Autodesk Inventor part; units mm, degrees
ref_plane "Work Plane1" through (-0.254, 8.163, 9.525) normal (-1, 0, 0) x (0, 0, 1)
ref_plane "YZ Plane" through (0, 0, 0) normal (1, 0, 0) x (0, 1, 0)
ref_plane "XZ Plane" through (0, 0, 0) normal (0, 1, 0) x (-1, 0, 0)
sketch "Sketch1" plane through (0, 0, 0) normal (0, 0, 1) x (1, 0, 0)
  line L0 (0, 0) -> (66.675, 0)
  line L1 (66.675, 0) -> (66.675, 12.9255)
  line L2 (66.675, 12.9255) -> (0, 12.9255)
  line L3 (0, 12.9255) -> (0, 0)
  line L4 (66.675, 12.9255) -> (47.625, 12.9255)
  line L5 (47.625, 12.9255) -> (47.625, -23.7521)
  line L6 (47.625, -23.7521) -> (66.675, -23.7521)
  line L7 (66.675, -23.7521) -> (66.675, 12.9255)
  point P0 (57.15, -14.2271)
  point P1 (34.4424, 12.9255)
  point P2 (9.0424, 12.9255)
  dimension "d0" = 66.675
  dimension "d3" = 25.4
  dimension "d4" = 27.1526
  dimension "d5" = 0
  dimension "d41" = 48.1076
  dimension "d42" = 19.05
  dimension "d43" = 9.525
extrude "Extrusion1" add sketch "Sketch1" along normal blind 6.35
sketch "Sketch2" plane through (0, 0, 6.35) normal (0, 0, 1) x (1, 0, 0)
  line L0 (66.675, -23.7521) -> (66.675, 12.9255)
  line L1 (47.625, 0) -> (47.625, -23.7521)
  line L2 (66.675, 12.9255) -> (0, 12.9255)
  line L3 (47.625, -23.7521) -> (66.675, -23.7521)
  point P0 (0, 0)
  point P1 (57.15, -14.2271)
  dimension "d12" = 27.1526
  dimension "d44" = 9.525
  dimension "d45" = 9.525
  dimension "d46" = 9.525
hole "Hole1" at (57.15, -14.2271, 6.35) direction (0, 0, -1) diameter 6.25 depth 25.4 tip angle 118
sketch "Sketch3" plane through (0, 0, 6.35) normal (0, 0, 1) x (1, 0, 0)
  circle A0 centre (57.15, -14.2271) radius 3.125
  circle A1 centre (57.15, -14.2271) radius 9.525
  line L0 (47.625, -23.7521) -> (66.675, -23.7521)
  point P0 (0, 0)
extrude "Extrusion2" add sketch "Sketch3" along normal blind 12.7
fillet "Fillet1" radius 6.35 2 edges at (66.675, -23.7521, 3.175) (47.625, -23.7521, 3.175)
fillet "Fillet2" radius 25.4 2 edges at (47.625, 0, 3.175) (66.675, 12.9255, 3.175)
sketch "Sketch4" plane through (0, 0, 6.35) normal (0, 0, 1) x (1, 0, 0)
  line L0 (0, 12.9255) -> (0, 0)
  line L1 (0, 12.9255) -> (40.7924, 12.9255)
  line L2 (40.7924, 12.9255) -> (40.7924, 8.163)
  line L3 (40.7924, 8.163) -> (0, 8.163)
  line L4 (0, 8.163) -> (0, 12.9255)
  circle A0 centre (57.15, -14.2271) radius 3.125
  dimension "d24" = 16.3576
  dimension "d25" = 4.7625
extrude "Extrusion3" add sketch "Sketch4" along normal blind 9.525 contours L1 L2 L3 L0
fillet "Fillet3" radius 6.35 2 edges at (40.7924, 10.5443, 15.875) (0, 10.5443, 15.875)
fillet "Fillet4" radius 6.35 1 edges at (40.7924, 10.5443, 6.35)
sketch "Sketch5" plane through (6.35, 8.163, 15.875) normal (0, -1, 0) x (1, 0, 0)
  line L0 (47.675, 3.175) -> (53.925, 3.175)
  point P0 (-6.35, -15.875)
  point P1 (2.6924, -5.0739)
  point P2 (28.0924, -5.0739)
  point P3 (50.8, 3.175)
  dimension "d30" = 25.4
  dimension "d31" = 22.7076
hole "Hole2" at (9.0424, 8.163, 10.8011) at (34.4424, 8.163, 10.8011) at (57.15, 8.163, 19.05) direction (0, 1, 0) diameter 4.4958 depth 25.4 tip angle 118
fillet "Fillet5" radius 6.35 1 edges at (0, 0, 3.175)
fillet "Fillet6" radius 3.175 1 edges at (47.625, -14.2271, 19.05)
fillet "Fillet7" radius 3.175 1 edges at (54.025, -14.2271, 19.05)
ref_plane "Work Plane1" through (-0.254, 8.163, 9.525) normal (-1, 0, 0) x (0, 0, 1)
properties part number "supporty"
Check sheet for the modelled part. Datum: model origin and axes. Units: mm. A direction names the side the tool comes from. Round coordinates to 2 decimals unless told otherwise and drop trailing zeros. Write each loop counter-clockwise with the first axis right and the second up, starting at its lowest first coordinate (ties: lowest second). Pieces come first, ordered by that corner, then holes. Notation, with made-up numbers: (-14.75, 51) -> (7.25, 51) arc R22 cw to (7.25, 58) -> close; hole circle Ø5 at (58.25, 31.5). An arc over 180 degrees is marked (long way). One line per question, with ' | ' between items. Start each with the question number.
1. Scan lines: line 1 along Y through (x, z) = (57.15, 7); line 2 along X through (y, z) = (11.5, 11.5); line 3 along Z through (x, y) = (23, 5). Record each from-to range of solid material in increasing order. Write a range as from..to.
2. Depth check by flat-ended pin: pin 1 (4 mm diameter, centred on x = 15.5, y = 10, fed in from +Z) (3 decimals); pin 2 (1 mm diameter, centred on x = 30.5, y = 1.5, fed in from -Z); pin 3 (1.5 mm diameter, centred on x = 45.5, y = 3, fed in from +Z); pin 4 (4 mm diameter, centred on x = 34.44, z = 10.8, fed in from +Y). Enter the tip coordinate at first touch or a pass-through.
3. Release check for a two-part mould opening along Z. For faces 6 (the face through (32.55, 10.58, 9.59)), 7 (the face through (11.037, 10.578, 9.764)), 8 (the face through (38, 1, 6.35)), 9 (the face through (66.675, -15, 3)) record: +Z half, -Z half, draft (parallel to the pull), parting line (faces both ways), or undercut.
4. Sectioned sample at A-A, the plane z = 7. Count the separate pieces of the cut face and the enclosed holes in it, then the cut area to 3 significant figures.
5. Sectioned sample at B-B, the plane x = 35.5. Record the cut outline in (y, z), then the cut area to 3 significant figures.
6. Set-up check for faces 1 (the face through (19, 8.163, 11)), 2 (the face through (64, -21.1, 6.35)), 3 (the face through (15, 0, 3)), 4 (the face through (20, 11, 15.875)), 5 (the face through (64.765, -21.941, 3.219)): record each of +Z, -Z, +X, -X, +Y, -Y from which the full face is reachable in a straight line by a thin tool's end or side.
Taken from the geometry:
1) line 1: y = -23.75..-17.35, -11.1..-4.7 | line 2: x = 0.31..6.91, 11.18..32.31, 36.58..40.48 | line 3: z = 0..6.35
2) pin 1: stops at z = 15.875 | pin 2: stops at z = 0 | pin 3: stops at z = 6.35 | pin 4: passes through
3) face 6: undercut | face 7: undercut | face 8: +Z half | face 9: draft
4) separate pieces: 2 | enclosed holes: 1 | area: 463 mm^2
5) outline: (-3.15, 0) -> (12.93, 0) -> (12.93, 8.82) -> (8.16, 8.82) -> (8.16, 6.35) -> (-3.15, 6.35) -> close; (8.16, 12.78) -> (12.93, 12.78) -> (12.93, 15.79) -> (8.16, 15.79) -> close | area: 128 mm^2
6) face 1: +Z, +X, -X, -Y | face 2: +Z, +X, -Y | face 3: +Z, -Z, -X, -Y | face 4: +Z, +X, -X, +Y, -Y | face 5: +Z, -Z, +X, -Y
